from build123d import *

# Parameters (mm, degrees)
F1_DEPTH = 445
F2_W     = 680
F2_H     = 400
F3_DEPTH = 86.1864572875
F4_W     = 75
F4_H     = 1450
F5_DEPTH = 180.001


with BuildPart() as f1:
    # F0 (on Right) → F1 (new body, symmetric)
    with BuildSketch(Plane.YZ):
        Polygon((0, 180), (0, 0), (2070, 0), (1848.4551352237, 1256.4433638354), (1898.4544831016, 1256.6987298108), (1898.4544831016, 1281.6987298108), (1959.0762613666, 1316.6987298108), (1934.0762613666, 1360), (1587.6660998528, 1160), (1129.0381352408, 1119.8752523205), (1129.0381352408, 1069.8752523205), (1729.0381352408, 1069.8752523205), (1885.9471516896, 180), align=None)
    extrude(amount=F1_DEPTH, both=True)

    # F2 (on face) → F3 (cut, up to face)
    with BuildSketch(Plane(origin=(0, -88.6558352853, 1013.3408342556), x_dir=(1, 0, 0), z_dir=(0, -0.0871557427, 0.9961946981))):
        with Locations((-5, 1422.3453636709)):
            Rectangle(F2_W, F2_H)
    extrude(amount=-F3_DEPTH, mode=Mode.SUBTRACT)

    # F4 (on face) → F5 (cut, through all)
    with BuildSketch(Plane.XY.offset(180)):
        with Locations((-407.5, 725)):
            Rectangle(F4_W, F4_H)
        with Locations((407.5, 725)):
            Rectangle(F4_W, F4_H)
    extrude(amount=-F5_DEPTH, mode=Mode.SUBTRACT)


solid = f1.part
For this review, take the finished solid that the model builds, in its own axes (mm). A direction names the side the tool comes from. Round coordinates to 2 decimals unless told otherwise and drop trailing zeros. Write each loop counter-clockwise with the first axis right and the second up, starting at its lowest first coordinate (ties: lowest second). Pieces come first, ordered by that corner, then holes. Notation, with made-up numbers: (-34, 22) -> (18, 22) arc R29 cw to (18, 58) -> close; hole circle Ø11 at (84, 12). An arc over 180 degrees is marked (long way). Put each result on its own line as item: value.
Q1. Consider section D-D on z = 115. State the section outline as (x, y) points.
Determined:
outline: (-445, 1450) -> (-370, 1450) -> (-370, 0) -> (370, 0) -> (370, 1450) -> (445, 1450) -> (445, 2049.72) -> (-445, 2049.72) -> close
Q2. Consider section C-C on y = 1266.5. State the section outline as (x, z) points.
Determined:
outline: (-445, 1069.88) -> (-345, 1069.88) -> (-345, 1131.9) -> (-445, 1131.9) -> close; (-370, 0) -> (370, 0) -> (370, 180) -> (-370, 180) -> close; (335, 1069.88) -> (445, 1069.88) -> (445, 1131.9) -> (335, 1131.9) -> close
Q3. Consider section A-A on x = 200. State the section outline as (y, z) points, and give its area (3 significant figures).
Determined:
outline: (0, 0) -> (2070, 0) -> (1848.46, 1256.44) -> (1898.45, 1256.7) -> (1898.45, 1281.7) -> (1959.08, 1316.7) -> (1934.08, 1360) -> (1587.67, 1160) -> (1527.52, 1154.74) -> (1534.94, 1069.88) -> (1729.04, 1069.88) -> (1885.95, 180) -> (0, 180) -> close; (1129.04, 1069.88) -> (1133.41, 1069.88) -> (1129.04, 1119.88) -> close
area: 563,000 mm^2
Q4. To check wall thickness, follow L1, parallel to Z at x = 238.5, y = 1341; L2, parallel to X at y = 539.5, z = 118; L3, parallel to Y at x = 195.5, z = 1090. State the ranges of each line that lie inside material, in increasing order. Write a range as [from, to].
Determined:
L1: z = [0, 180]
L2: x = [-370, 370]
L3: y = [1129.04, 1131.65], [1533.18, 1877.8]
Q5. Machinability: for faces 4 (the flat face through (6, 956, 180)), 5 (the flat face through (6, 1129.038, 1095)), 6 (the flat face through (-9.76, 1531.176, 1112.9)), which of the approach directions +Z, -Z, +X, -X, +Y, -Y give a long, thin tool a straight path to every point of the face, cutting with its end or side? Answer none if there is none.
Determined:
face 4: +X, -X, -Y
face 5: +Z, +X, -X, -Y
face 6: none
Q6. The part is to be moulded in two halves that separate along X. For faces 1 (the flat face through (6.23, 1806.394, 631.167)), 2 (the flat face through (-345, 1328, 1105)), 3 (the flat face through (-445, 1841, 582)), say which applies: released by +X, released by -X, zero draft, split by the parting line, or undercut.
Determined:
face 1: zero draft
face 2: undercut
face 3: released by -X
Q7. Consider section B-B on y = 1659.5. State the section outline as (x, z) points.
Determined:
outline: (-445, 0) -> (445, 0) -> (445, 180) -> (-445, 180) -> close; (-445, 1069.88) -> (445, 1069.88) -> (445, 1201.47) -> (-445, 1201.47) -> close
Q8. Clearance check with flat-ended pins moving along their axes: pin 1 Ø25 at (x, z) = (61.5, 1093.5) entering from -Y; pin 2 Ø6 at (x, y) = (336.5, 296.5) entering from +Z; pin 3 Ø22.5 at (x, z) = (-415.5, 97) entering from -Y. State where each tip first meets the part, or that it passes through.
Determined:
pin 1: stops at y = 1129.04
pin 2: stops at z = 180
pin 3: stops at y = 1450
